Here's how the part is built. I have some questions about the finished solid (model axes, mm). A direction names the side the tool comes from. Give positions to 0.01 mm unless a question says otherwise; leave off trailing zeros. Write each loop counter-clockwise with the first axis right and the second up, starting at its lowest first coordinate (ties: lowest second). Pieces come first, ordered by that corner, then holes. Notation, with made-up numbers: (76, -8.5) -> (85, -8.5) arc R19 ccw to (85, 16.5) -> close; hole circle Ø5 at (-11.75, -38.75). An arc over 180 degrees is marked (long way). Put each result on its own line as item: value. Start each with the question number.
from build123d import *

# Parameters (mm, degrees)
F0_R     = 4.25
F0_R_2   = 2.75
F1_DEPTH = 3
F2_DEPTH = 8.5


# Not quite as in the source:
# - a feature names something its author has since deleted; it is built from what else it names


with BuildPart() as f1:
    # F0 (on Top) → F1 (new body)
    with BuildSketch(Plane.XY):
        with BuildLine():
            ThreePointArc((-20.0475404255, -5.1050880284), (-14.4143064726, -4.9130538455), (-11.6516802209, 0))
            ThreePointArc((-11.6516802209, 0), (-13.7942703105, 4.4776214376), (-18.6252780431, 5.6183011996))
            ThreePointArc((-18.6252780431, 5.6183011996), (-23.1017631579, 0.7560122426), (-20.0475404255, -5.1050880284))
        make_face()
        with Locations((-17.4016802209, 0)):
            Circle(F0_R, mode=Mode.SUBTRACT)
        with BuildLine():
            ThreePointArc((-18.6252780431, 5.6183011996), (-13.7942703105, 4.4776214376), (-11.6516802209, 0))
            ThreePointArc((-11.6516802209, 0), (-14.4143064726, -4.9130538455), (-20.0475404255, -5.1050880284))
            Line((-20.0475404255, -5.1050880284), (13.6632948995, -38.0643911727))
            ThreePointArc((13.6632948995, -38.0643911727), (16.8311240547, -29.8688761508), (24.3801958358, -34.3647768698))
            Line((24.3801958358, -34.3647768698), (31.8937613277, 22.2850285764))
            ThreePointArc((31.8937613277, 22.2850285764), (23.4337103416, 19.9124465773), (22.5117964167, 28.6503915729))
            Line((22.5117964167, 28.6503915729), (-18.6252780431, 5.6183011996))
        make_face()
        Polygon((14.6992403306, -23.6933170767), (-8.2995714993, -1.2072290356), (19.7657026362, 14.5061375255), align=None, mode=Mode.SUBTRACT)
        with BuildLine():
            ThreePointArc((32.3347594316, 25.6100088156), (28.3621582746, 30.1635639823), (22.5117964167, 28.6503915729))
            ThreePointArc((22.5117964167, 28.6503915729), (23.4337103416, 19.9124465773), (31.8937613277, 22.2850285764))
            Line((31.8937613277, 22.2850285764), (32.3347594316, 25.6100088156))
        make_face()
        with Locations((26.6620065254, 24.670660922)):
            Circle(F0_R, mode=Mode.SUBTRACT)
        with BuildLine():
            ThreePointArc((24.3801958358, -34.3647768698), (16.8311240547, -29.8688761508), (13.6632948995, -38.0643911727))
            Line((13.6632948995, -38.0643911727), (16.0615827249, -40.4092127917))
            ThreePointArc((16.0615827249, -40.4092127917), (20.5837618045, -40.7393733758), (23.9391977319, -37.6897571089))
            Line((23.9391977319, -37.6897571089), (24.3801958358, -34.3647768698))
        make_face()
        with Locations((18.7074429296, -35.3041247633)):
            Circle(F0_R, mode=Mode.SUBTRACT)
        with Locations((-17.4016802209, 0)):
            Circle(F0_R)
        with Locations((-17.4016802209, 0)):
            Circle(F0_R_2, mode=Mode.SUBTRACT)
        with Locations((26.6620065254, 24.670660922)):
            Circle(F0_R)
        with Locations((26.6620065254, 24.670660922)):
            Circle(F0_R_2, mode=Mode.SUBTRACT)
        with Locations((18.7074429296, -35.3041247633)):
            Circle(F0_R)
        with Locations((18.7074429296, -35.3041247633)):
            Circle(F0_R_2, mode=Mode.SUBTRACT)
    extrude(amount=F1_DEPTH)

    # F0 (on Top) → F2 (join)
    with BuildSketch(Plane.XY):
        with Locations((26.6620065254, 24.670660922)):
            Circle(F0_R)
        with Locations((26.6620065254, 24.670660922)):
            Circle(F0_R_2, mode=Mode.SUBTRACT)
        with Locations((-17.4016802209, 0)):
            Circle(F0_R)
        with Locations((-17.4016802209, 0)):
            Circle(F0_R_2, mode=Mode.SUBTRACT)
        with Locations((18.7074429296, -35.3041247633)):
            Circle(F0_R)
        with Locations((18.7074429296, -35.3041247633)):
            Circle(F0_R_2, mode=Mode.SUBTRACT)
    extrude(amount=F2_DEPTH)


solid = f1.part
1) Thinking about a two-plate mould opening in X: for faces 1 (the flat face through (-2.246, -22.51, 1.479)), 2 (the flat face through (-17, -3, 8.5)), 3 (the flat face through (17.268, -4.326, 1.479)), which applies, released by +X, released by -X, zero draft, split by the parting line, or undercut?
2) I'm going to push flat-ended pins straight in: pin 1 Ø1 at (x, z) = (25, 2) entering from +Y; pin 2 Ø3 at (x, z) = (8, 2) entering from -Y. Where does each tip first touch, or does it pass through?
3) I want a section at D-D, the plane z = 1.25. Write out the boundary of the cut face in (x, y).
4) I want a section at A-A, the plane z = 6.5. Write out the boundary of the cut face in (x, y), and give its area (3 significant figures).
5) Which directions (+Z, -Z, +X, -X, +Y, -Y) give clear straight access to the entire face, cutting with the end or side of a thin tool? Please do faces 4 (the cylindrical face through (23.289, 22.085, 5.712)), 5 (the flat face through (3.361, -12.608, 1.479)), 6 (the cylindrical face through (28.447, 30.137, 1.479)).
6) I want a section at C-C, the plane x = 1.5. Write out the boundary of the cut face in (y, z), and give its area (3 significant figures).
7) I need wall thicknesses on probe 1 along Y at (x, z) = (26.5, 4.5); probe 2 along Y at (x, z) = (-17.5, 8.25); probe 3 along Z at (x, y) = (28, 13.5). Which ranges of each line are inside material? Lowest first, please.
8) I want a section at B-B, the plane y = -10.5. Write out the boundary of the cut face in (x, z).
Established:
1. face 1: released by -X
1. face 2: zero draft
1. face 3: undercut
2. pin 1: stops at y = 30.3
2. pin 2: stops at y = -33.99
3. outline: (-20.05, -5.11) -> (16.06, -40.41) arc R5.75 ccw to (23.94, -37.69) -> (32.33, 25.61) arc R5.75 ccw to (22.51, 28.65) -> (-18.63, 5.62) arc R5.75 ccw to start; hole circle Ø5.5 at (-17.4, 0); hole (-8.3, -1.21) -> (14.7, -23.69) -> (19.77, 14.51) -> close; hole circle Ø5.5 at (18.71, -35.3); hole circle Ø5.5 at (26.66, 24.67)
4. outline: circle Ø8.5 at (-17.4, 0); circle Ø8.5 at (18.71, -35.3); circle Ø8.5 at (26.66, 24.67); hole circle Ø5.5 at (-17.4, 0); hole circle Ø5.5 at (18.71, -35.3); hole circle Ø5.5 at (26.66, 24.67)
4. area: 99.0 mm2
5. face 4: +Z
5. face 5: +Z, -Z
5. face 6: +Z, -Z, +Y
6. outline: (-26.17, 0) -> (-10.79, 0) -> (-10.79, 3) -> (-26.17, 3) -> close; (4.28, 0) -> (16.89, 0) -> (16.89, 3) -> (4.28, 3) -> close
6. area: 84.0 mm2
7. probe 1: y = 20.42 to 21.93, 27.42 to 28.92
7. probe 2: y = -4.25 to -2.75, 2.75 to 4.25
7. probe 3: z = 0 to 3
8. outline: (-14.53, 0) -> (1.21, 0) -> (1.21, 3) -> (-14.53, 3) -> close; (16.45, 0) -> (27.55, 0) -> (27.55, 3) -> (16.45, 3) -> close
